```python
from build123d import *

# Parameters (mm, degrees)
PAD_DEPTH    = 45
POCKET_DEPTH = 40


with BuildPart() as part:
    # Sketch → Pad (new body)
    with BuildSketch(Plane.XY):
        Polygon((13.380021, 13.380021), (0, 0), (13.380021, -13.380021), (18.339621, -12.5), (25, -12.5), (25, 12.5), (18.339621, 12.5), align=None)
    extrude(amount=PAD_DEPTH)

    # Sketch001 (on Face9 of Pad) → Pocket (cut)
    with BuildSketch(Plane.XY.offset(45)):
        Polygon((25, 9.302202), (22, 9.302202), (22, 10.5), (17.5, 10.5), (17.5, -10.5), (22, -10.5), (22, -9.302202), (25, -9.302202), align=None)
    extrude(amount=-POCKET_DEPTH, mode=Mode.SUBTRACT)


solid = part.part
```
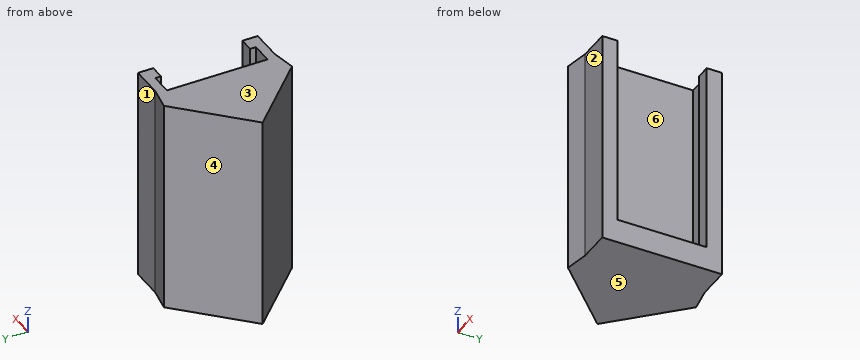
Part model, mm, in its own coordinate system. Face numbers are marked on the shaded views. A direction names the side the tool comes from. Round coordinates to 2 decimals unless told otherwise and drop trailing zeros. Write each loop counter-clockwise with the first axis right and the second up, starting at its lowest first coordinate (ties: lowest second). Pieces come first, ordered by that corner, then holes. Notation, with made-up numbers: M 1,-32.5 L 35,-32.5 A14 ccw 35,-7.5 Z; hole C 31,86 d1. An arc over 180 degrees is marked long. Answer as CSV lines item,"result". Start each with the question number.
1) Band-saw the part on C-C (y = 2). List the corners of the cut face in (x, z), then the cut area to 3 significant figures.
2) Drop flat-ended pins along their axis: pin 1 (8 mm diameter, centred on y = 9, z = 8.5, fed in from +X); pin 2 (3.5 mm diameter, centred on x = 20.5, z = 30.5, fed in from -Y); pin 3 (3.5 mm diameter, centred on x = 21.5, z = 16.5, fed in from +Y); pin 4 (2 mm diameter, centred on x = 21.5, y = -2, fed in from +Z). Give the stop position or say it passes through.
3) Which spindle directions (+Z, -Z, +X, -X, +Y, -Y) get a long thin tool onto all of the face, cutting with end or side? Do the marked faces 1, 2 and 3. Say none if no direction does.
4) Band-saw the part on B-B (x = 20). List the corners of the cut face in (y, z).
5) Band-saw the part on D-D (y = 4.75). List the corners of the cut face in (x, z), then the cut area to 3 significant figures.
6) Band-saw the part on A-A (z = 6). List the corners of the cut face in (x, y), then the cut area to 3 significant figures.
7) Mould opens along Y. For the marked faces 4, 5 and 6 say: +Y half, -Y half, draft (parallel to the pull), parting line (faces both ways), or undercut.
8) Drill centre lines: L1, parallel to Y at x = 21.25, z = 30.5; L2, parallel to Y at x = 22.25, z = 32.5; L3, parallel to Z at x = 19.5, y = -0.75. Where is each one in solid material? Low to high.
Worked out:
1,outline,"M 2,0 L 25,0 L 25,5 L 17.5,5 L 17.5,45 L 2,45 Z"
1,area,"735 mm²"
2,pin 1,"x = 25"
2,pin 2,"y = -12.5"
2,pin 3,"y = 12.5"
2,pin 4,"z = 5"
3,face 1,"+Z, -Z, +X, +Y"
3,face 2,"+Z, -Z, +X, -Y"
3,face 3,"+Z, +X, -X, +Y, -Y"
4,outline,"M -12.5,0 L 12.5,0 L 12.5,45 L 10.5,45 L 10.5,5 L -10.5,5 L -10.5,45 L -12.5,45 Z"
5,outline,"M 4.75,0 L 25,0 L 25,5 L 17.5,5 L 17.5,45 L 4.75,45 Z"
5,area,"611 mm²"
6,outline,"M 0,0 L 13.38,-13.38 L 18.34,-12.5 L 25,-12.5 L 25,-9.3 L 22,-9.3 L 22,-10.5 L 17.5,-10.5 L 17.5,10.5 L 22,10.5 L 22,9.3 L 25,9.3 L 25,12.5 L 18.34,12.5 L 13.38,13.38 Z"
6,area,"324 mm²"
7,face 4,"+Y half"
7,face 5,"draft"
7,face 6,"undercut"
8,L1,"-12.5 to -10.5, 10.5 to 12.5"
8,L2,"-12.5 to -9.3, 9.3 to 12.5"
8,L3,"0 to 5"
